Source: three-view drawing plus pictorial views. Frame: mm from the lowest corner of the part. A direction names the side the tool comes from. Give positions to 0.01 mm unless a question says otherwise; leave off trailing zeros. Write each loop counter-clockwise with the first axis right and the second up, starting at its lowest first coordinate (ties: lowest second). Pieces come first, ordered by that corner, then holes. Notation, with made-up numbers: (19.25, -21.75) -> (45.25, -21.75) arc R30 ccw to (45.25, 6.25) -> close; hole circle Ø9 at (58.5, -24). An arc over 180 degrees is marked (long way). Use a Markdown table: item, result. Add a question column.
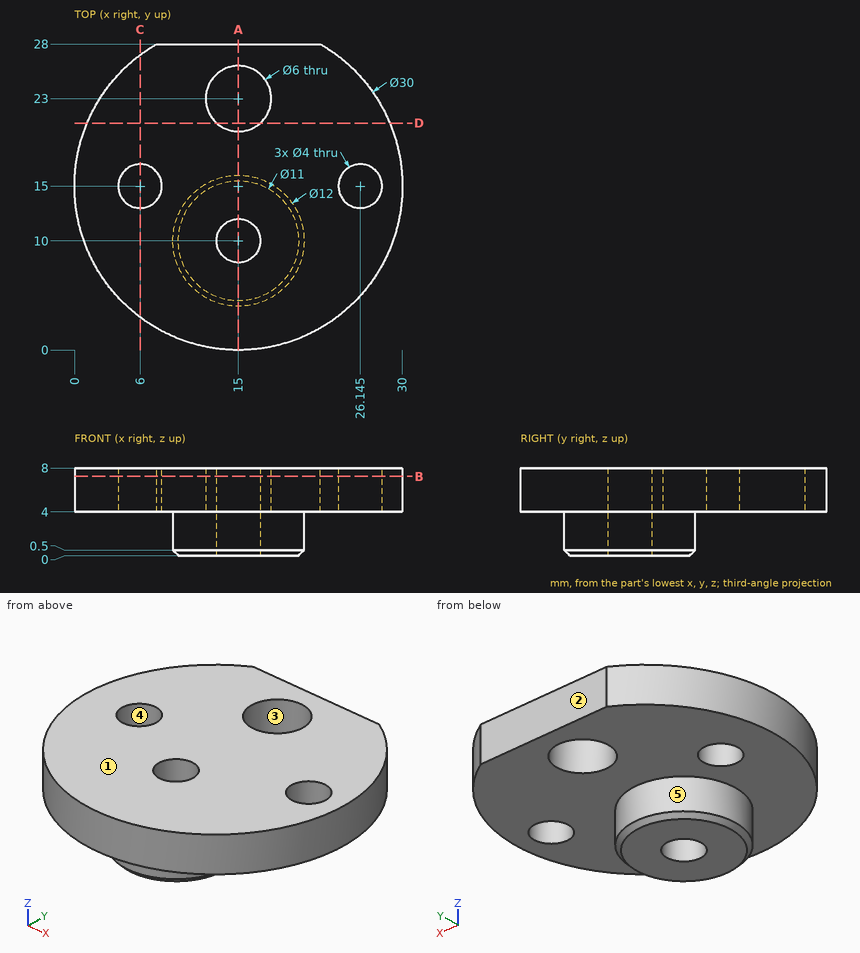
(1) Cut plane C-C on x = 6. Return the cut outline in (y, z).
(2) Material intervals for L1, parallel to Y at x = 15, z = 6.9; L2, parallel to Z at x = 21.5, y = 2.75; L3, parallel to X at y = 16.75, z = 5.75, sorted ascending.
(3) Mould query, pull axis Y, two halves, no side actions, for the marked faces 1, 2 and 3. Classes: +Y half, -Y half, draft (parallel to the pull), parting line (faces both ways), or undercut.
(4) First-contact query: pin 1 Ø2 at (y, z) = (11, 5.5) entering from +X. Flat tip, straight axial feed; report the tip coordinate or a pass-through.
(5) Cut plane D-D on y = 20.75. Return the cut outline in (x, z).
(6) Cut plane B-B on z = 7.25. Return the cut outline in (x, y) (3 decimals), then the cut area to 3 significant figures.
(7) Access query for the marked faces 4 and 5. Directions: +Z, -Z, +X, -X, +Y, -Y. A direction counts if a zero-diameter tool reaches every point of the face in a straight line with its end or side. Return the directions, or none.
(8) Cut plane A-A on x = 15. Return the cut outline in (y, z), then the cut area to 3 significant figures.
Output:
| question | item | result |
|---|---|---|
| 1 | outline | (3, 4) -> (13, 4) -> (13, 8) -> (3, 8) -> close; (17, 4) -> (27, 4) -> (27, 8) -> (17, 8) -> close |
| 2 | L1 | 0 to 8, 12 to 20, 26 to 28 |
| 2 | L2 | 4 to 8 |
| 2 | L3 | 0.1 to 5.03, 6.97 to 25.18, 27.11 to 29.9 |
| 3 | face 1 | draft |
| 3 | face 2 | +Y half |
| 3 | face 3 | undercut |
| 4 | pin 1 | x = 29.7 |
| 5 | outline | (1.15, 4) -> (13.02, 4) -> (13.02, 8) -> (1.15, 8) -> close; (16.98, 4) -> (28.85, 4) -> (28.85, 8) -> (16.98, 8) -> close |
| 6 | outline | (7.517, 28) arc R15 ccw (long way) to (22.483, 28) -> close; hole circle Ø4 at (6, 15); hole circle Ø6 at (15, 23); hole circle Ø4 at (15, 10); hole circle Ø4 at (26.145, 15) |
| 6 | area | 621 mm^2 |
| 7 | face 4 | +Z, -Z |
| 7 | face 5 | -Z |
| 8 | outline | (0, 4) -> (4, 4) -> (4, 0.5) -> (4.5, 0) -> (8, 0) -> (8, 8) -> (0, 8) -> close; (12, 0) -> (15.5, 0) -> (16, 0.5) -> (16, 4) -> (20, 4) -> (20, 8) -> (12, 8) -> close; (26, 4) -> (28, 4) -> (28, 8) -> (26, 8) -> close |
| 8 | area | 104 mm^2 |
